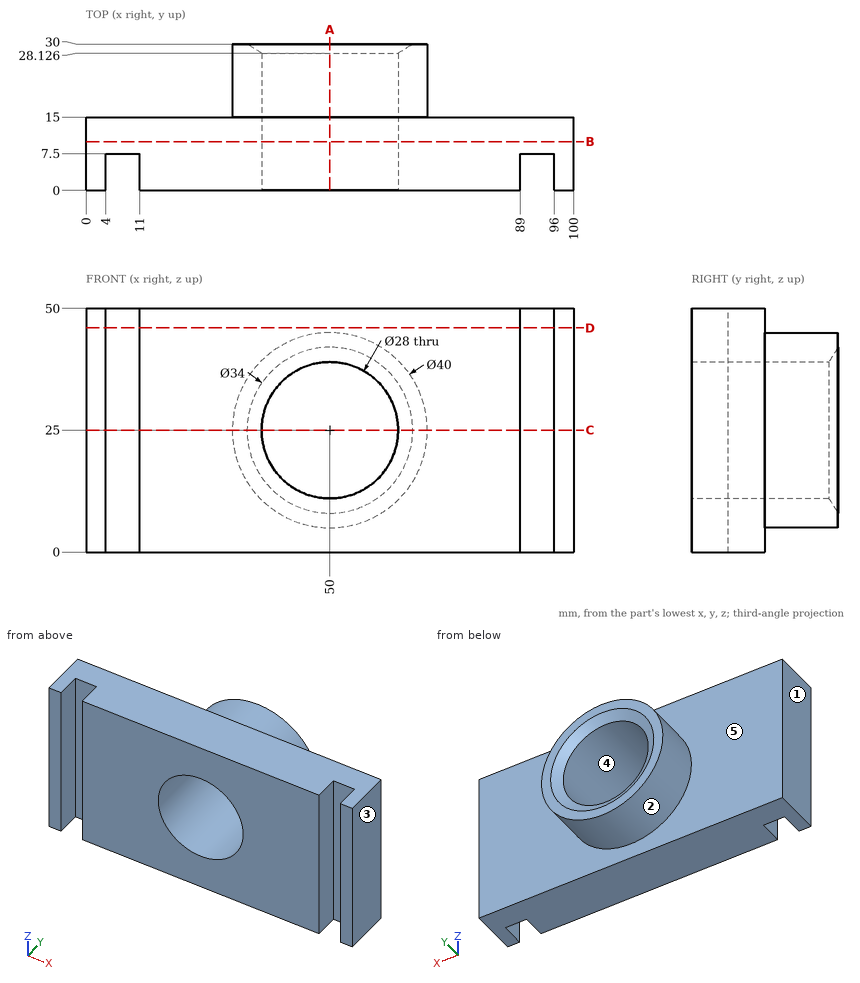
Geometry check sheet. Reference: drawing and pictorial views, mm from the part's lowest x, y, z. A direction names the side the tool comes from. Round coordinates to 2 decimals unless told otherwise and drop trailing zeros. Order: outer loops, then holes, each group sorted by start corner. A loop starts at its lowest first (then second) coordinate and runs counter-clockwise, first axis right, second up. Notation, with made-up numbers: (75, -2.5) - (89, -2.5) arc R10 ccw to (89, 9.5) - close; hole circle Ø11 at (25, 46). An arc over 180 degrees is marked (long way). One line per question, with ' | ' between items. Start each with the question number.
(1) Thickness scan on L1, parallel to X at y = 7, z = 35.5; L2, parallel to X at y = 13, z = 25; L3, parallel to Y at x = 73.5, z = 23. Record the ranges inside material, lowest first. Write a range as [from, to].
(2) Access from +Z, -Z, +X, -X, +Y, -Y to the whole of each face (thin tool, end or side, straight path). Record for the marked faces 1 and 2.
(3) Sectioned sample at B-B on y = 10. Record the cut outline in (x, z), and give its area (3 significant figures).
(4) Sectioned sample at C-C on z = 25. Record the cut outline in (x, y).
(5) Sectioned sample at A-A on x = 50. Record the cut outline in (y, z), and give its area (3 significant figures).
(6) Depth check by flat-ended pin: pin 1 Ø12 at (x, z) = (20, 15.5) entering from -Y; pin 2 Ø10 at (x, z) = (82.5, 12) entering from +Y; pin 3 Ø10 at (y, z) = (24, 6) entering from +X; pin 4 Ø3.5 at (x, z) = (7.5, 19.5) entering from -Y. Enter the tip coordinate at first touch or a pass-through.
(7) Release check for a two-part mould opening along X. For the marked faces 3, 4 and 5 record: released by +X, released by -X, zero draft, split by the parting line, or undercut.
(8) Sectioned sample at D-D on z = 46. Record the cut outline in (x, y), and give its area (4 significant figures).
Conclusion:
1) L1: x = [0, 4], [11, 40.74], [59.26, 89], [96, 100] | L2: x = [0, 36], [64, 100] | L3: y = [0, 15]
2) face 1: +Z, -Z, -X, +Y, -Y | face 2: +Y
3) outline: (0, 0) - (100, 0) - (100, 50) - (0, 50) - close; hole circle Ø28 at (50, 25) | area: 4,380 mm2
4) outline: (0, 0) - (4, 0) - (4, 7.5) - (11, 7.5) - (11, 0) - (36, 0) - (36, 28.13) - (33, 30) - (30, 30) - (30, 15) - (0, 15) - close; (64, 0) - (89, 0) - (89, 7.5) - (96, 7.5) - (96, 0) - (100, 0) - (100, 15) - (70, 15) - (70, 30) - (67, 30) - (64, 28.13) - close
5) outline: (0, 0) - (15, 0) - (15, 5) - (30, 5) - (30, 8) - (28.13, 11) - (0, 11) - close; (0, 39) - (28.13, 39) - (30, 42) - (30, 45) - (15, 45) - (15, 50) - (0, 50) - close | area: 504 mm2
6) pin 1: stops at y = 0 | pin 2: stops at y = 15 | pin 3: stops at x = 64.28 | pin 4: stops at y = 7.5
7) face 3: released by +X | face 4: undercut | face 5: zero draft
8) outline: (0, 0) - (4, 0) - (4, 7.5) - (11, 7.5) - (11, 0) - (89, 0) - (89, 7.5) - (96, 7.5) - (96, 0) - (100, 0) - (100, 15) - (0, 15) - close | area: 1,395 mm2
